from build123d import *

# Parameters (mm, degrees)
SKETCH_R         = 2
EXTRUDE_DEPTH    = 2
SKETCH001_R      = 0.75
HOLE_DEPTH       = 3.001
SKETCH002_W      = 3
SKETCH002_H      = 3
REVOLUTION_ANGLE = -180


with BuildPart() as part:
    # Sketch → Extrude (new body, symmetric)
    with BuildSketch(Plane.XY):
        Polygon((-4, 5), (4, 5), (4, -5), (-4, -5), (-19, -5), (-19, -2), (-12, -2), align=None)
        Circle(SKETCH_R, mode=Mode.SUBTRACT)
    extrude(amount=EXTRUDE_DEPTH, both=True)

    # Sketch001 (on Face6 of Extrude) → Hole (cut, through all)
    with BuildSketch(Plane(origin=(0, -2, 0), x_dir=(-1, 0, 0), z_dir=(0, 1, 0))):
        with Locations((15, 0)):
            Circle(SKETCH001_R)
    extrude(amount=-HOLE_DEPTH, mode=Mode.SUBTRACT)

    # Sketch002 (on Face4 of Hole) → Revolution (revolve)
    with BuildSketch(Plane(origin=(0, 0, -2), x_dir=(1, 0, 0), z_dir=(0, 0, -1))):
        with Locations((-20.5, 3.5)):
            Rectangle(SKETCH002_W, SKETCH002_H)
    revolve(axis=Axis((-15, -5, -2), (0, -1, 0)), revolution_arc=REVOLUTION_ANGLE)


solid = part.part
Verification items for the finished model (mm, model axes). Give positions to 0.01 mm unless a question says otherwise; leave off trailing zeros. Order: outer loops, then holes, each group sorted by start corner. A loop starts at its lowest first (then second) coordinate and runs counter-clockwise, first axis right, second up. Notation, with made-up numbers: M 59.25,15.25 L 81.25,15.25 A11 ccw 81.25,35.25 Z; hole C 39,61.25 d3. An arc over 180 degrees is marked long. Answer as a JSON object with one key per item and string values. Group by question number.
1) Scan lines: line 1 along Z through (x, y) = (-15, -3.35); line 2 along Y through (x, z) = (0, -1.15); line 3 along Y through (x, z) = (-14.75, -1). Record each from-to range of solid material in increasing order. Write a range as [from, to].
2) Cross-section at D-D (z = 1.75). Enter the section's corners in (x, y).
3) Cross-section at C-C (z = -0.5). Enter the section's corners in (x, y).
4) Mould release check, pull along X, two halves, no side actions. Record for faces 1 (the face through (-8.06, 1.45, 0.03)), 2 (the face through (-14.25, -3.48, 0.03)), 3 (the face through (-2, -1, 2)), 4 (the face through (-17.21, -3.52, 4.64)): released by +X, released by -X, zero draft, split by the parting line, or undercut.
5) Cross-section at A-A (x = 0). Enter the section's corners in (y, z), then the cut area to 3 significant figures.
6) Depth check by flat-ended pin: pin 1 Ø4.5 at (x, y) = (0, 0) entering from +Z; pin 2 Ø0.9 at (x, z) = (-15, 0) entering from -Y; pin 3 Ø4 at (x, z) = (-5.5, 3) entering from +Y; pin 4 Ø1 at (y, z) = (-3.5, -1) entering from -X. Enter the tip coordinate at first touch or a pass-through.
7) Cross-section at B-B (y = 0). Enter the section's corners in (x, z), then the cut area to 3 significant figures.
Result sheet:
{
 "1": {"line 1": "z = [-2, -0.75], [0.75, 5]", "line 2": "y = [-5, -2], [2, 5]", "line 3": "y = [-5, -2]"},
 "2": {"outline": "M -20.91,-5 L 4,-5 L 4,5 L -4,5 L -12,-2 L -20.91,-2 Z; hole C 0,0 d4"},
 "3": {"outline": "M -21.84,-5 L -15.56,-5 L -15.56,-2 L -21.84,-2 Z; M -14.44,-5 L 4,-5 L 4,5 L -4,5 L -12,-2 L -14.44,-2 Z; hole C 0,0 d4"},
 "4": {"face 1": "released by -X", "face 2": "undercut", "face 3": "zero draft", "face 4": "split by the parting line"},
 "5": {"outline": "M -5,-2 L -2,-2 L -2,2 L -5,2 Z; M 2,-2 L 5,-2 L 5,2 L 2,2 Z", "area": "24.0 mm2"},
 "6": {"pin 1": "stops at z = 2", "pin 2": "passes through", "pin 3": "stops at y = 5", "pin 4": "stops at x = -21.98"},
 "7": {"outline": "M -9.71,-2 L -2,-2 L -2,2 L -9.71,2 Z; M 2,-2 L 4,-2 L 4,2 L 2,2 Z", "area": "38.9 mm2"}
}
